Source: three-view drawing plus pictorial views. Frame: mm from the lowest corner of the part. A direction names the side the tool comes from. Give positions to 0.01 mm unless a question says otherwise; leave off trailing zeros. Order: outer loops, then holes, each group sorted by start corner. A loop starts at its lowest first (then second) coordinate and runs counter-clockwise, first axis right, second up.
1) Section B-B, the plane z = 5.5. Return loops of the section in (x, y), plus the area to 3 significant figures.
2) Access query for the marked faces 1, 2 and 3. Directions: +Z, -Z, +X, -X, +Y, -Y. A direction counts if a zero-diameter tool reaches every point of the face in a straight line with its end or side. Return the directions, or none.
3) First-contact query: P1, Ø2.5, axis at x = 43.5, y = 16.5, coming from the -Z side; P2, Ø11, axis at y = 8, z = 31, coming from the -X side; P3, Ø3, axis at x = 75, z = 5.5, coming from the +Y side; P4, Ø6.5, axis at x = 38, y = 3.5, coming from the -Z side. Flat tips, straight axial feed; report the tip coordinate or a pass-through.
4) Draft query along X for the marked faces 4, 5 and 6. Return one class per face: released by +X, released by -X, zero draft, split by the parting line, or undercut.
5) Section A-A, the plane x = 75. Return loops of the section in (y, z).
6) Section C-C, the plane z = 29.5. Return loops of the section in (x, y).
7) Section D-D, the plane x = 54. Return loops of the section in (y, z), plus the area to 3 significant figures.
8) Material intervals for line 1 (Z direction, x = 75, y = 23.45); line 2 (X direction, y = 7, z = 32); line 3 (Y direction, x = 68, z = 5), sorted ascending.
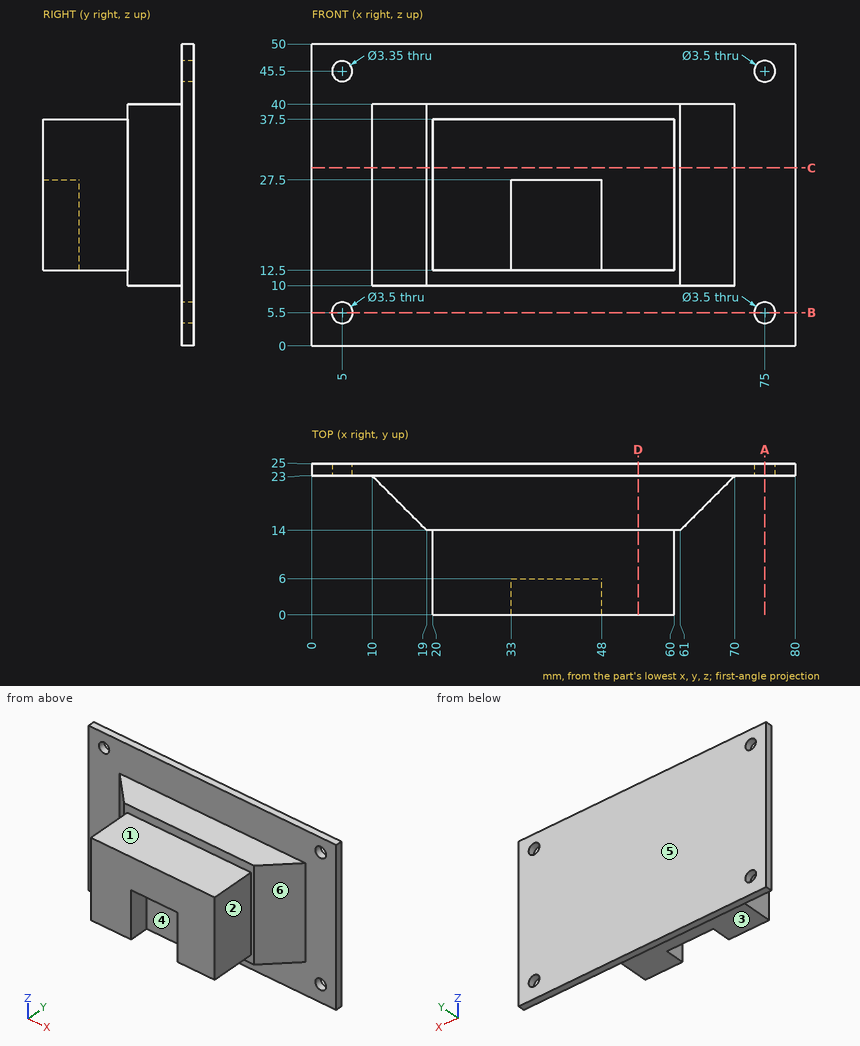
From the geometry:
1. outline: (0, 23) - (3.25, 23) - (3.25, 25) - (0, 25) - close; (6.75, 23) - (73.25, 23) - (73.25, 25) - (6.75, 25) - close; (76.75, 23) - (80, 23) - (80, 25) - (76.75, 25) - close
1. area: 146 mm2
2. face 1: +Z, +X, -X, -Y
2. face 2: +Z, -Z, +X, -Y
2. face 3: -Z, +X, -X, -Y
3. P1: stops at z = 10
3. P2: stops at x = 20
3. P3: passes through
3. P4: stops at z = 12.5
4. face 4: undercut
4. face 5: zero draft
4. face 6: released by +X
5. outline: (23, 0) - (25, 0) - (25, 3.75) - (23, 3.75) - close; (23, 7.25) - (25, 7.25) - (25, 43.75) - (23, 43.75) - close; (23, 47.25) - (25, 47.25) - (25, 50) - (23, 50) - close
6. outline: (0, 23) - (10, 23) - (19, 14) - (20, 14) - (20, 0) - (60, 0) - (60, 14) - (61, 14) - (70, 23) - (80, 23) - (80, 25) - (0, 25) - close
7. outline: (0, 12.5) - (14, 12.5) - (14, 10) - (23, 10) - (23, 0) - (25, 0) - (25, 50) - (23, 50) - (23, 40) - (14, 40) - (14, 37.5) - (0, 37.5) - close
7. area: 720 mm2
8. line 1: z = 0 to 3.75, 7.25 to 43.75, 47.25 to 50
8. line 2: x = 20 to 60
8. line 3: y = 23 to 25
